Can you work these out from the model? Positions are in its coordinate system, mm. A direction names the side the tool comes from. Coordinates: 2 decimals unless noted, no trailing zeros. Order: outer loops, then holes, each group sorted by start corner. A loop starts at its lowest first (then second) coordinate and runs counter-clockwise, first axis right, second up. Notation, with made-up numbers: (73, 8.25) -> (93, 8.25) arc R23 ccw to (93, 40.25) -> close; hole circle Ø8 at (78.5, -31.75). An arc over 180 degrees is marked (long way). Use a Markdown table: item, result. Add a question column.
1. If I drill on line 1 along Z through (x, y) = (0, 26); line 2 along Y through (x, z) = (0.5, -7.5); line 3 along Y through (x, z) = (5.5, 3), over which ranges is the centre line in solid material (lowest first)? Write a range as from..to.
2. Suppose I cut it at C-C, the plane y = -1. List the corners of the cut face in (x, z) for me, then the cut area to 3 significant figures.
3. For faces 1 (the cylindrical face through (0.325, 25.549, 7.536)), 2 (the cylindrical face through (-3.755, 14.297, -11.923)), which set-ups out of +Z, -Z, +X, -X, +Y, -Y let a thin tool reach every point of the face, with its end or its side?
4. Suppose I cut it at D-D, the plane z = 5. List the corners of the cut face in (x, y) for me, then the cut area to 3 significant figures.
5. We'd pull the mould along Z, two halves only. Please class faces 3 (the flat face through (0, 22, 9)), 4 (the flat face through (6, -5.5, 0)), 5 (the flat face through (0, 22, -9)), 6 (the cylindrical face through (9.173, -2.712, -0.705)): pulls with the +Z half, pulls with the -Z half, needs draft (parallel to the pull), parting line crosses it, or undercut.
6. Suppose I cut it at B-B, the plane x = 0. List the corners of the cut face in (y, z) for me.
7. For pin 1 Ø1.5 at (y, z) = (20, -5.5) entering from +X; pin 2 Ø1.5 at (x, z) = (-6.5, 0.5) entering from -Y; pin 3 Ø6 at (x, z) = (3.5, -1) entering from +Y; pin 4 Ø3.5 at (x, z) = (0, -9) entering from +Y, each with a flat end and sliding along its axis, tell me the tip position at first contact or that it passes through.
8. Suppose I cut it at A-A, the plane z = 0. List the corners of the cut face in (x, y) for me.
```python
from build123d import *

# Parameters (mm, degrees)
SKETCH_1_R          = 12.5
EXTRUDE_3_DEPTH     = 29
SKETCH_4_R          = 6
EXTRUDE_4_DEPTH     = 2
SKETCH_5_R          = 2
EXTRUDE_5_DEPTH     = 10
SKETCH_6_R          = 1.5
CUT_EXTRUDE_1_DEPTH = 19
SKETCH_7_R          = 3.25
EXTRUDE_6_DEPTH     = 5.5


with BuildPart() as part:
    # 草图1 → 凸台-拉伸3 (new body)
    with BuildSketch(Plane(origin=(0, 0, 0), x_dir=(0, 0, -1), z_dir=(0, 1, 0))):
        Circle(SKETCH_1_R)
    extrude(amount=EXTRUDE_3_DEPTH)

    # 草图4 → 凸台-拉伸4 (add)
    with BuildSketch(Plane(origin=(0, 29, 0), x_dir=(0, 0, -1), z_dir=(0, 1, 0))):
        with Locations(Location((0, 0, 0), (0, 0, 90))):
            Circle(SKETCH_4_R)
    extrude(amount=EXTRUDE_4_DEPTH)

    # 草图5 → 凸台-拉伸5 (add)
    with BuildSketch(Plane(origin=(0, 31, 0), x_dir=(0, 0, -1), z_dir=(0, 1, 0))):
        with Locations(Location((0, 0, 0), (0, 0, 90))):
            Circle(SKETCH_5_R)
    extrude(amount=EXTRUDE_5_DEPTH)

    # 草图6 → 切除-拉伸1 (cut)
    with BuildSketch(Plane(origin=(0, 41, 0), x_dir=(0, 0, -1), z_dir=(0, 1, 0))):
        with Locations(Location((-9, 0, 0), (0, 0, 90))):
            Circle(SKETCH_6_R)
        with Locations(Location((9, 0, 0), (0, 0, 90))):
            Circle(SKETCH_6_R)
    extrude(amount=-CUT_EXTRUDE_1_DEPTH, mode=Mode.SUBTRACT)

    # 草图7 → 凸台-拉伸6 (add)
    with BuildSketch(Plane(origin=(0, 0, 0), x_dir=(0, 0, 1), z_dir=(0, -1, 0))):
        with Locations((0, -6)):
            Circle(SKETCH_7_R)
    extrude(amount=EXTRUDE_6_DEPTH)


solid = part.part
```
Worked out:
| question | item | result |
|---|---|---|
| 1 | line 1 | z = -12.5..-10.5, -7.5..7.5, 10.5..12.5 |
| 1 | line 2 | y = 0..29 |
| 1 | line 3 | y = -5.5..29 |
| 2 | outline | circle Ø6.5 at (6, 0) |
| 2 | area | 33.2 mm² |
| 3 | face 1 | +Y |
| 3 | face 2 | +Y, -Y |
| 4 | outline | (-11.46, 0) -> (11.46, 0) -> (11.46, 29) -> (3.32, 29) -> (3.32, 31) -> (-3.32, 31) -> (-3.32, 29) -> (-11.46, 29) -> close |
| 4 | area | 678 mm² |
| 5 | face 3 | undercut |
| 5 | face 4 | needs draft |
| 5 | face 5 | undercut |
| 5 | face 6 | parting line crosses it |
| 6 | outline | (0, -12.5) -> (29, -12.5) -> (29, -10.5) -> (22, -10.5) -> (22, -7.5) -> (29, -7.5) -> (29, -6) -> (31, -6) -> (31, -2) -> (41, -2) -> (41, 2) -> (31, 2) -> (31, 6) -> (29, 6) -> (29, 7.5) -> (22, 7.5) -> (22, 10.5) -> (29, 10.5) -> (29, 12.5) -> (0, 12.5) -> close |
| 7 | pin 1 | stops at x = 11.56 |
| 7 | pin 2 | stops at y = 0 |
| 7 | pin 3 | stops at y = 41 |
| 7 | pin 4 | stops at y = 29 |
| 8 | outline | (-12.5, 0) -> (2.75, 0) -> (2.75, -5.5) -> (9.25, -5.5) -> (9.25, 0) -> (12.5, 0) -> (12.5, 29) -> (6, 29) -> (6, 31) -> (2, 31) -> (2, 41) -> (-2, 41) -> (-2, 31) -> (-6, 31) -> (-6, 29) -> (-12.5, 29) -> close |
